Autodesk Inventor part; units mm, degrees
ref_plane "YZ Plane" through (0, 0, 0) normal (1, 0, 0) x (0, 1, 0)
ref_plane "XZ Plane" through (0, 0, 0) normal (0, 1, 0) x (-1, 0, 0)
ref_plane "XY Plane" through (0, 0, 0) normal (0, 0, 1) x (1, 0, 0)
sketch "Sketch1" plane through (0, 0, 0) normal (0, 0, 1) x (1, 0, 0)
  line L0 (-38.1, -31.75) -> (38.1, -31.75)
  line L1 (38.1, -31.75) -> (38.1, 31.75)
  line L2 (38.1, 31.75) -> (-38.1, 31.75)
  line L3 (-38.1, 31.75) -> (-38.1, -31.75)
  line L4 (-38.1, -31.75) -> (38.1, 31.75) construction
  line L5 (38.1, -31.75) -> (-38.1, 31.75) construction
  point P0 (0, 0)
  dimension "d0" = 76.2
  dimension "d1" = 63.5
extrude "Extrusion1" add sketch "Sketch1" along normal blind 1.5875
sketch "Sketch2" plane through (0, 0, 1.5875) normal (0, 0, 1) x (1, 0, 0)
  line L0 (0, -44.45) -> (0, 44.45)
  line L1 (-53.34, 0) -> (53.34, 0)
  line L2 (38.1, 31.75) -> (-38.1, 31.75)
  point P0 (0, 0)
  point P1 (-29.765, 22.225)
  point P2 (29.765, 22.225)
  point P3 (29.765, -22.225)
  point P4 (-29.765, -22.225)
  dimension "d4" = 59.53
  dimension "d5" = 9.525
hole "Hole1" at (-29.765, -22.225, 1.5875) at (-29.765, 22.225, 1.5875) at (29.765, 22.225, 1.5875) at (29.765, -22.225, 1.5875) direction (0, 0, -1) diameter 4.7752 end through all
sketch "Sketch4" plane through (0, 0, 1.5875) normal (0, 0, 1) x (1, 0, 0)
  line L0 (38.1, 31.75) -> (-38.1, 31.75)
  line L1 (-23.8125, -31.75) -> (23.8125, -31.75)
  line L2 (23.8125, -31.75) -> (23.8125, 31.75)
  line L3 (23.8125, 31.75) -> (-23.8125, 31.75)
  line L4 (-23.8125, 31.75) -> (-23.8125, -31.75)
  line L5 (-23.8125, -31.75) -> (23.8125, 31.75) construction
  line L6 (23.8125, -31.75) -> (-23.8125, 31.75) construction
  point P0 (0, 0)
  point P1 (-23.8125, 31.75)
  dimension "d13" = 47.625
extrude "Extrusion2" add sketch "Sketch4" along normal blind 6.35
sketch "Sketch5" plane through (-38.1, -31.75, 0) normal (0, -1, 0) x (1, 0, 0)
  line L0 (76.2, 0) -> (0, 0)
  line L1 (15.875, 7.1437) -> (60.325, 7.1437)
  line L2 (60.325, 7.1437) -> (60.325, 0)
  line L3 (60.325, 0) -> (15.875, 0)
  line L4 (15.875, 0) -> (15.875, 7.1437)
  line L5 (14.2875, 7.9375) -> (61.9125, 7.9375)
  line L6 (14.2875, 1.5875) -> (14.2875, 7.9375)
  line L7 (61.9125, 1.5875) -> (61.9125, 7.9375)
  point P0 (38.1, 0)
  dimension "d16" = 0.7937
  dimension "d17" = 1.5875
  dimension "d18" = 1.5875
extrude "Extrusion3" cut sketch "Sketch5" along normal through all both and the other way through all
sketch "Sketch6" plane through (0, 0, 7.9375) normal (0, 0, 1) x (1, 0, 0)
  line L0 (-16, -23.8125) -> (-16, 23.8125) construction
  line L1 (-15, -23.8125) -> (-15, 23.8125)
  line L2 (-17, 23.8125) -> (-17, -23.8125)
  arc A0 (-17, -23.8125) -> (-15, -23.8125) centre (-16, -23.8125) ccw
  arc A1 (-15, 23.8125) -> (-17, 23.8125) centre (-16, 23.8125) ccw
  line L3 (16, -23.8125) -> (16, 23.8125) construction
  line L4 (15, -23.8125) -> (15, 23.8125)
  line L5 (17, 23.8125) -> (17, -23.8125)
  arc A2 (15, -23.8125) -> (17, -23.8125) centre (16, -23.8125) ccw
  arc A3 (17, 23.8125) -> (15, 23.8125) centre (16, 23.8125) ccw
  line L6 (0, -44.45) -> (0, 44.45)
  line L7 (-53.34, 0) -> (53.34, 0)
  line L8 (23.8125, 31.75) -> (-23.8125, 31.75)
  point P0 (0, 0)
  point P1 (-16, 0)
  point P2 (16, 0)
  dimension "d21" = 32
  dimension "d22" = 2
  dimension "d23" = 7.9375
extrude "Extrusion4" cut sketch "Sketch6" against normal through all
fillet "Fillet1" radius 3.175 4 edges at (-38.1, 31.75, 0.7937) (-38.1, -31.75, 0.7937) (38.1, -31.75, 0.7937) (38.1, 31.75, 0.7937)
fillet "Fillet2" radius 4.7625 2 edges at (-22.225, 0, 7.1437) (22.225, 0, 7.1437)
properties part number "RC_CAR_LIDAR_PLATE"
Input: part model. Units: mm. Frame: model coordinates. A direction names the side the tool comes from. Give positions to 0.01 mm unless a question says otherwise; leave off trailing zeros. Order: outer loops, then holes, each group sorted by start corner. A loop starts at its lowest first (then second) coordinate and runs counter-clockwise, first axis right, second up. Notation, with made-up numbers: (67, 15) - (103, 15) arc R26 ccw to (103, 51) - close; hole circle Ø9 at (80, 33.5). An arc over 180 degrees is marked (long way). Answer as a JSON object with one key per item and string values. Group by question number.
Q1. Cut plane A-A, the plane x = 16. Output: boundary loops of the cut face in (y, z).
Q2. Line query: probe 1 along X at (y, z) = (22.5, 1.5) (3 decimals); probe 2 along X at (y, z) = (-12.5, 7.25); probe 3 along X at (y, z) = (23, 2) (1 decimal). Output: solid intervals per line, ascending.
Q3. Cut plane B-B, the plane z = 5.25. Output: boundary loops of the cut face in (x, y), then the cut area to 3 significant figures.
Q4. Mould query, pull axis Y, two halves, no side actions, for faces 6 (the face through (-0.2, -31.75, 7.5)), 7 (the face through (-31.379, 23.985, 0.783)), 8 (the face through (-31, 0, 1.588)), 9 (the face through (37.19, 30.8, 0.8)). Classes: pulls with the +Y half, pulls with the -Y half, needs draft (parallel to the pull), parting line crosses it, or undercut.
Q5. Cut plane D-D, the plane x = -21. Output: boundary loops of the cut face in (y, z).
Q6. Set-up query: faces 1 (the face through (-23.812, 0, 5)), 2 (the face through (22.225, 0, 1)), 3 (the face through (27.4, 22.54, 0.78)), 4 (the face through (37.15, -30.84, 0.8)), 5 (the face through (31, 0, 1.588)). Return all of +Z, -Z, +X, -X, +Y, -Y with unobstructed straight access to the full face (end or side cutting, diameter ignored); none if empty.
Q7. Cut plane C-C, the plane x = 25. Output: boundary loops of the cut face in (y, z).
Q8. First-contact query: pin 1 Ø1.5 at (y, z) = (2.5, 4.5) entering from +X; pin 2 Ø7.5 at (x, y) = (-29.765, -22.225) entering from -Z; pin 3 Ø11.5 at (x, y) = (-30, 12.5) entering from +Z; pin 4 Ø0.9 at (y, z) = (0, 7.5) entering from -X. Flat tips, straight axial feed; report the tip coordinate or a pass-through.
Results:
{
 "1": {"outline": "(-31.75, 7.14) - (-24.81, 7.14) - (-24.81, 7.94) - (-31.75, 7.94) - close; (24.81, 7.14) - (31.75, 7.14) - (31.75, 7.94) - (24.81, 7.94) - close"},
 "2": {"probe 1": "-38.1 to -32.137, -27.393 to -22.225, 22.225 to 27.393, 32.137 to 38.1", "probe 2": "-23.81 to -17, -15 to 15, 17 to 23.81", "probe 3": "-23.8 to -22.2, 22.2 to 23.8"},
 "3": {"outline": "(-23.81, -31.75) - (-21.26, -31.75) - (-21.26, 31.75) - (-23.81, 31.75) - close; (21.26, -31.75) - (23.81, -31.75) - (23.81, 31.75) - (21.26, 31.75) - close", "area": "324 mm^2"},
 "4": {"face 6": "pulls with the -Y half", "face 7": "undercut", "face 8": "needs draft", "face 9": "pulls with the +Y half"},
 "5": {"outline": "(-31.75, 5.57) - (31.75, 5.57) - (31.75, 7.94) - (-31.75, 7.94) - close"},
 "6": {"face 1": "+Z, -X, +Y, -Y", "face 2": "-Z, +Y, -Y", "face 3": "+Z, -Z", "face 4": "+Z, -Z, +X, -Y", "face 5": "+Z, +X, +Y, -Y"},
 "7": {"outline": "(-31.75, 0) - (31.75, 0) - (31.75, 1.59) - (-31.75, 1.59) - close"},
 "8": {"pin 1": "x = 23.81", "pin 2": "z = 0", "pin 3": "z = 1.59", "pin 4": "x = -23.81"}
}
